from build123d import *

# Parameters (mm, degrees)
F1_DEPTH = 50


# Not quite as in the source:
# - a feature names something its author has since deleted; it is built from what else it names


with BuildPart() as f1:
    # F0 (on Top) → F1 (new body)
    with BuildSketch(Plane.XY):
        Polygon((-28, 24.552706346), (-28, 0), (0, 0), (0, 24.552706346), (-9.2052005051, 24.552706346), align=None)
        with BuildLine():
            Line((-28, 46.552706346), (-28, 24.552706346))
            Line((-28, 24.552706346), (-9.2052005051, 24.552706346))
            Line((-9.2052005051, 24.552706346), (-9.2052005051, 31.202706346))
            ThreePointArc((-9.2052005051, 31.202706346), (-7.3453285656, 35.6928344065), (-2.8552005051, 37.552706346))
            Line((-2.8552005051, 37.552706346), (28.8586538925, 37.552706346))
            Line((28.8586538925, 37.552706346), (42.7064734879, 37.552706346))
            Line((42.7064734879, 37.552706346), (42.7064734879, 46.552706346))
            Line((42.7064734879, 46.552706346), (-28, 46.552706346))
        make_face()
        with BuildLine():
            ThreePointArc((28.8586538925, 37.552706346), (35.7825636902, 35), (42.7064734879, 37.552706346))
            Line((42.7064734879, 37.552706346), (28.8586538925, 37.552706346))
        make_face()
        with BuildLine():
            ThreePointArc((-21.0234507531, 52.8717201964), (-25.9128577435, 51.2591427749), (-28, 46.552706346))
            Line((-28, 46.552706346), (42.7064734879, 46.552706346))
            Line((42.7064734879, 46.552706346), (-21.0234507531, 52.8717201964))
        make_face()
        Polygon((0, 0), (-28, 0), (-28, -24.552706346), (-9.2052005051, -24.552706346), (0, -24.552706346), align=None)
        with BuildLine():
            Line((-9.2052005051, -24.552706346), (-28, -24.552706346))
            Line((-28, -24.552706346), (-28, -46.552706346))
            Line((-28, -46.552706346), (42.7064734879, -46.552706346))
            Line((42.7064734879, -46.552706346), (42.7064734879, -37.552706346))
            Line((42.7064734879, -37.552706346), (28.8586538925, -37.552706346))
            Line((28.8586538925, -37.552706346), (-2.8552005051, -37.552706346))
            ThreePointArc((-2.8552005051, -37.552706346), (-7.3453285656, -35.6928344065), (-9.2052005051, -31.202706346))
            Line((-9.2052005051, -31.202706346), (-9.2052005051, -24.552706346))
        make_face()
        with BuildLine():
            Line((42.7064734879, -46.552706346), (-28, -46.552706346))
            ThreePointArc((-28, -46.552706346), (-25.9128577435, -51.2591427749), (-21.0234507531, -52.8717201964))
            Line((-21.0234507531, -52.8717201964), (42.7064734879, -46.552706346))
        make_face()
        with BuildLine():
            Line((28.8586538925, -37.552706346), (42.7064734879, -37.552706346))
            ThreePointArc((42.7064734879, -37.552706346), (35.7825636902, -35), (28.8586538925, -37.552706346))
        make_face()
    extrude(amount=F1_DEPTH)


solid = f1.part
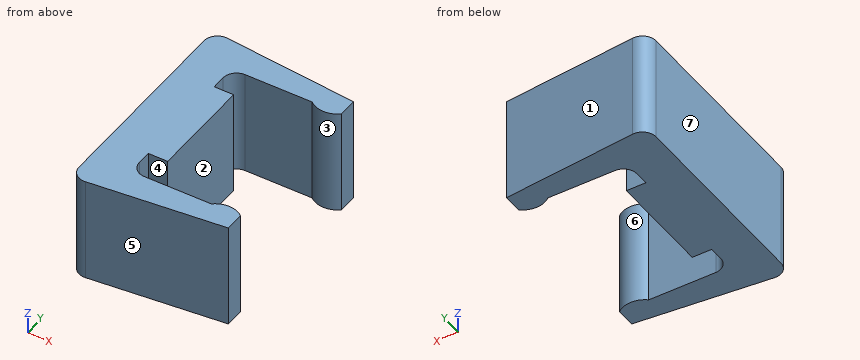
Could you check a few things on this model? Use its own coordinates, in mm. Face numbers are marked on the shaded views. A direction names the side the tool comes from. Give positions to 0.01 mm unless a question says otherwise; leave off trailing zeros. Order: outer loops, then holes, each group sorted by start corner. A loop starts at its lowest first (then second) coordinate and runs counter-clockwise, first axis right, second up. Notation, with made-up numbers: (53, -34) - (109, -34) arc R23 cw to (109, -3) - close; hole circle Ø11 at (20.25, -16.5). An arc over 180 degrees is marked (long way). One line per item, written item: value. Start each with the question number.
1. Imagine slicing it at C-C on y = -28. List the corners of the cut face in (x, z) for me, plus the area to 3 significant figures.
2. Imagine slicing it at B-B on z = 13. List the corners of the cut face in (x, y) for me.
3. If I drill on probe 1 along Y at (x, z) = (-4, 20); probe 2 along X at (y, z) = (25, 2); probe 3 along Y at (x, z) = (-6, 24.5), over which ranges is the centre line in solid material (lowest first)?
4. Thinking about a two-plate mould opening in X: for the marked faces 4, 5, 6 and 7, which applies, +X half, -X half, draft (parallel to the pull), parting line (faces both ways), or undercut?
5. Imagine slicing it at D-D on x = 8.5. List the corners of the cut face in (y, z) for me, plus the area to 3 significant figures.
6. For P1, Ø24.5, axis at y = 1, z = 27.5, coming from the +X side; P2, Ø4.5, axis at x = -3, z = 17, coming from the -Y side; P3, Ø5, axis at y = -31, z = 17, coming from the +X side, each with a flat end and sliding along its axis, tell me the tip position at first contact or that it passes through.
7. For the marked faces 1, 2 and 3, which set-ups out of +Z, -Z, +X, -X, +Y, -Y let a thin tool reach every point of the face, with its end or its side?
8. Imagine slicing it at A-A on x = 23. List the corners of the cut face in (y, z) for me.
Values:
1. outline: (-28, 0) - (-9.21, 0) - (-9.21, 50) - (-28, 50) - close
1. area: 940 mm²
2. outline: (-28, -46.55) arc R6.35 ccw to (-21.02, -52.87) - (42.71, -46.55) - (42.71, -37.55) arc R10.67 ccw to (28.86, -37.55) - (-2.86, -37.55) arc R6.35 cw to (-9.21, -31.2) - (-9.21, -24.55) - (0, -24.55) - (0, 24.55) - (-9.21, 24.55) - (-9.21, 31.2) arc R6.35 cw to (-2.86, 37.55) - (28.86, 37.55) arc R10.67 ccw to (42.71, 37.55) - (42.71, 46.55) - (-21.02, 52.87) arc R6.35 ccw to (-28, 46.55) - close
3. probe 1: -51.18 to -37.45, -24.55 to 24.55, 37.45 to 51.18
3. probe 2: -28 to -9.21
3. probe 3: -51.38 to -36.72, -24.55 to 24.55, 36.72 to 51.38
4. face 4: draft
4. face 5: +X half
4. face 6: undercut
4. face 7: -X half
5. outline: (-49.94, 0) - (-37.55, 0) - (-37.55, 50) - (-49.94, 50) - close; (37.55, 0) - (49.94, 0) - (49.94, 50) - (37.55, 50) - close
5. area: 1,240 mm²
6. P1: x = 0
6. P2: y = -51.31
6. P3: x = -8.78
7. face 1: +Z, -Z, +X, +Y
7. face 2: +Z, -Z, +X
7. face 3: +Z, -Z
8. outline: (-48.51, 0) - (-37.55, 0) - (-37.55, 50) - (-48.51, 50) - close; (37.55, 0) - (48.51, 0) - (48.51, 50) - (37.55, 50) - close
